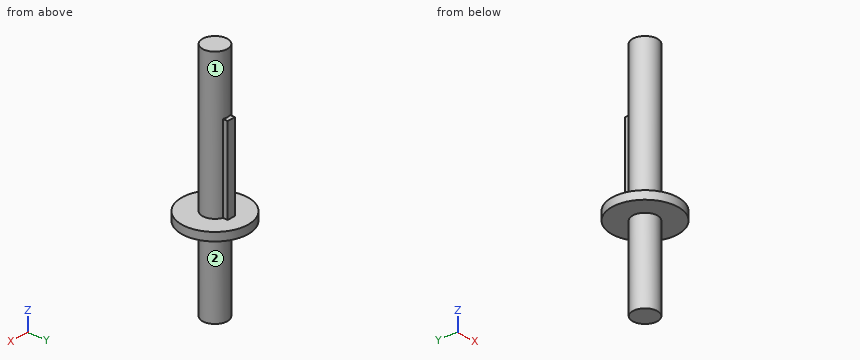
```python
from build123d import *

# Parameters (mm, degrees)
SKETCH1_R           = 3
BOSS_EXTRUDE1_DEPTH = 35
SKETCH3_R           = 8
BOSS_EXTRUDE3_DEPTH = 2
SKETCH2_W           = 2
SKETCH2_H           = 1.17
BOSS_EXTRUDE4_DEPTH = 20.7
SKETCH4_R           = 3
BOSS_EXTRUDE5_DEPTH = 20


with BuildPart() as part:
    # Sketch1 → Boss-Extrude1 (new body)
    with BuildSketch(Plane.XY):
        Circle(SKETCH1_R)
    extrude(amount=BOSS_EXTRUDE1_DEPTH)

    # Sketch3 → Boss-Extrude3 (add)
    with BuildSketch(Plane(origin=(0, 0, 0), x_dir=(-1, 0, 0), z_dir=(0, 0, -1))):
        Circle(SKETCH3_R)
    extrude(amount=BOSS_EXTRUDE3_DEPTH)

    # Sketch2 → Boss-Extrude4 (add)
    with BuildSketch(Plane(origin=(0, 0, 0), x_dir=(-1, 0, 0), z_dir=(0, 0, -1))):
        with Locations((0, 3.413427125)):
            Rectangle(SKETCH2_W, SKETCH2_H)
    extrude(amount=-BOSS_EXTRUDE4_DEPTH)

    # Sketch4 → Boss-Extrude5 (add)
    with BuildSketch(Plane(origin=(0, 0, -2), x_dir=(-1, 0, 0), z_dir=(0, 0, -1))):
        Circle(SKETCH4_R)
    extrude(amount=BOSS_EXTRUDE5_DEPTH)


solid = part.part
```
Verification items for the finished model (mm, model axes). Face numbers are marked on the shaded views. A direction names the side the tool comes from. Round coordinates to 2 decimals unless told otherwise and drop trailing zeros. Write each loop counter-clockwise with the first axis right and the second up, starting at its lowest first coordinate (ties: lowest second). Pieces come first, ordered by that corner, then holes.
1. Section check B-B on y = 0. Enter the section's corners in (x, z).
2. Access from +Z, -Z, +X, -X, +Y, -Y to the whole of each face (thin tool, end or side, straight path). Record for the marked faces 1 and 2.
3. Scan lines: L1, parallel to Z at x = -3.75, y = 2; L2, parallel to X at y = 3.75, z = 6; L3, parallel to X at y = -0.25, z = -7.5. Record each from-to range of solid material in increasing order.
4. Section check A-A on x = 0. Enter the section's corners in (y, z), plus the area to 3 significant figures.
5. Section check C-C on z = -6. Enter the section's corners in (x, y).
6. Section check D-D on z = 11. Enter the section's corners in (x, y), plus the area to 3 significant figures.
7. Gauge pin test, flat ends, axial feed: P1, Ø5, axis at y = 0, z = 21, coming from the +X side; P2, Ø0.9, axis at y = 3.5, z = 6, coming from the -X side; P3, Ø1, axis at x = -0.5, z = 7.5, coming from the +Y side. Record the tip position at first contact, or that the pin passes through.
Answer:
1. outline: (-8, -2) - (-3, -2) - (-3, -22) - (3, -22) - (3, -2) - (8, -2) - (8, 0) - (3, 0) - (3, 35) - (-3, 35) - (-3, 0) - (-8, 0) - close
2. face 1: +Z
2. face 2: -Z
3. L1: z = -2 to 0
3. L2: x = -1 to 1
3. L3: x = -2.99 to 2.99
4. outline: (-8, -2) - (-3, -2) - (-3, -22) - (3, -22) - (3, -2) - (8, -2) - (8, 0) - (4, 0) - (4, 20.7) - (3, 20.7) - (3, 35) - (-3, 35) - (-3, 0) - (-8, 0) - close
4. area: 383 mm2
5. outline: circle Ø6 at (0, 0)
6. outline: (-1, 2.83) arc R3 ccw (long way) to (1, 2.83) - (1, 4) - (-1, 4) - close
6. area: 30.4 mm2
7. P1: stops at x = 3
7. P2: stops at x = -1
7. P3: stops at y = 4
